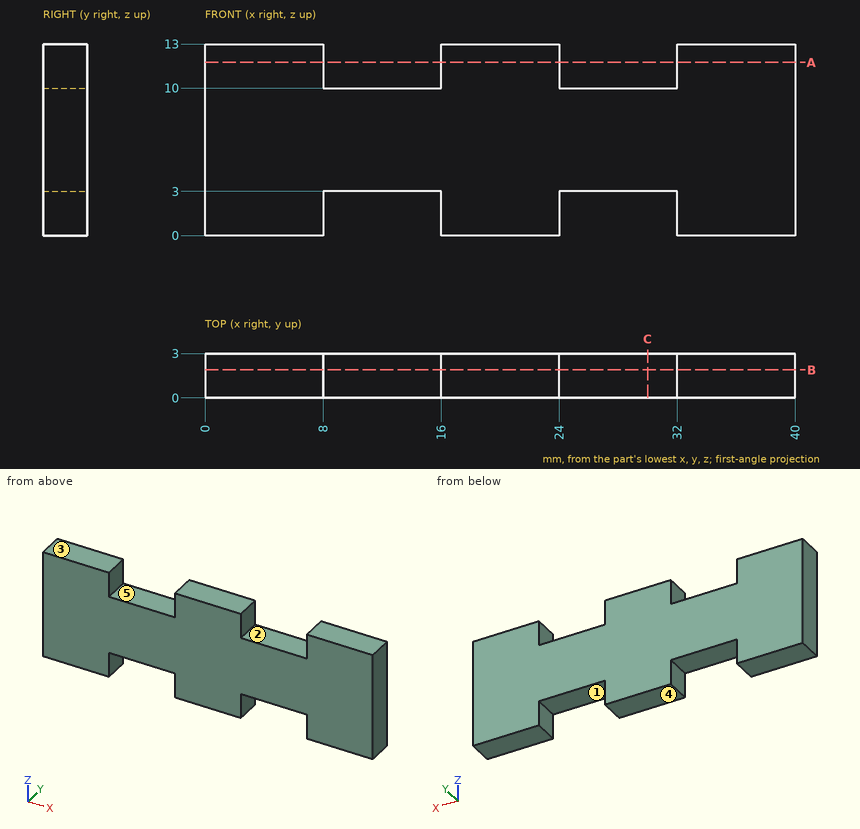
The drawing under review shows one solid part. Ordinate dimensions are in mm from its lowest x, y, z. A direction names the side the tool comes from. Round coordinates to 2 decimals unless told otherwise and drop trailing zeros. Loops run counter-clockwise (first coordinate to the right, second up) from the corner with the lowest first, then second, coordinate; pieces in that order, holes last. Notation, with made-up numbers: (60, 52) - (64, 52) arc R27 cw to (64, 74) - close; hole circle Ø3 at (-15, -20). An arc over 180 degrees is marked (long way). One line per item, written item: value. Start each with the question number.
1) For the marked faces 1, 2 and 3, list the 3-axis set-ups (+Z, -Z, +X, -X, +Y, -Y) from which the entire face can be reached by the end or side of a thin tool; tool diameter is ignored.
2) Consider section A-A on z = 11.75. Give the boundary of the cut face in (x, y).
3) To check wall thickness, follow L1, parallel to X at y = 2.35, z = 11; L2, parallel to Z at x = 30.5, y = 1. State the ranges of each line that lie inside material, in increasing order. Write a range as from..to.
4) Consider section C-C on x = 30. Give the boundary of the cut face in (y, z).
5) Insertion check: pin 1 Ø0.9 at (x, y) = (28, 2) entering from -Z. The pin has a flat end and moves straight along its axis. Give the tip position at first contact, or say it passes through.
6) Consider section B-B on y = 1.9. Give the boundary of the cut face in (x, z).
7) Draft analysis for pull direction X (two halves, no side actions). For the marked faces 4 and 5, state which applies: +X half, -X half, draft (parallel to the pull), parting line (faces both ways), or undercut.
Reported:
1. face 1: -Z, +Y, -Y
1. face 2: +Z, +Y, -Y
1. face 3: +Z, +X, -X, +Y, -Y
2. outline: (0, 0) - (8, 0) - (8, 3) - (0, 3) - close; (16, 0) - (24, 0) - (24, 3) - (16, 3) - close; (32, 0) - (40, 0) - (40, 3) - (32, 3) - close
3. L1: x = 0..8, 16..24, 32..40
3. L2: z = 3..10
4. outline: (0, 3) - (3, 3) - (3, 10) - (0, 10) - close
5. pin 1: stops at z = 3
6. outline: (0, 0) - (8, 0) - (8, 3) - (16, 3) - (16, 0) - (24, 0) - (24, 3) - (32, 3) - (32, 0) - (40, 0) - (40, 13) - (32, 13) - (32, 10) - (24, 10) - (24, 13) - (16, 13) - (16, 10) - (8, 10) - (8, 13) - (0, 13) - close
7. face 4: draft
7. face 5: undercut
